Could you check a few things on this model? Use its own coordinates, in mm. Face numbers are marked on the shaded views. A direction names the side the tool comes from. Round coordinates to 2 decimals unless told otherwise and drop trailing zeros. Write each loop counter-clockwise with the first axis right and the second up, starting at its lowest first coordinate (ties: lowest second). Pieces come first, ordered by that corner, then holes. Notation, with made-up numbers: (82, 78.25) -> (134, 78.25) arc R24 cw to (134, 97.25) -> close; hole circle Ø5 at (-12.5, -18.5). An arc over 180 degrees is marked (long way). Answer as CSV lines item,"result". Start each with the question number.
Q1. If I drill on line 1 (Z direction, x = 37, y = 35); line 2 (X direction, y = 33, z = 1.5); line 3 (Y direction, x = 20, z = 3.75), over which ranges is the centre line in solid material (lowest first)? Write a range as [from, to].
Q2. Imagine slicing it at B-B on y = 26. Please give me the cut outline in (x, z), and give its area (3 significant figures).
Q3. For the marked faces 1 and 2, which set-ups out of +Z, -Z, +X, -X, +Y, -Y let a thin tool reach every point of the face, with its end or its side?
Q4. Imagine slicing it at A-A on z = 1.75. Please give me the cut outline in (x, y).
Q5. Imagine slicing it at D-D on y = 3. Please give me the cut outline in (x, z), and give its area (3 significant figures).
Q6. Will these pins go through, and if not, where does the flat tip stop? pin 1 Ø1 at (y, z) = (32, 5) entering from -X; pin 2 Ø1.2 at (x, y) = (38.87, 51.02) entering from +Z; pin 3 Ø2.5 at (x, z) = (5.5, 1) entering from -Y; pin 4 Ø3.5 at (y, z) = (46.5, 1.5) entering from -X.
Q7. Imagine slicing it at C-C on x = 12.5. Please give me the cut outline in (y, z), and give its area (3 significant figures).
from build123d import *

# Parameters (mm, degrees)
SKETCH1_R           = 17.265633628
SKETCH1_R_2         = 1
SKETCH1_R_3         = 10
SKETCH1_W           = 25
SKETCH1_H           = 3
BOSS_EXTRUDE5_DEPTH = 3
SKETCH2_R           = 17.5
BOSS_EXTRUDE6_DEPTH = 6.5


with BuildPart() as part:
    # Sketch1 → Boss-Extrude5 (new body)
    # profile 1 of 3: a face of its own
    with BuildSketch(Plane.XY):
        with BuildLine():
            Line((0, 0), (7.5, 0))
            Line((7.5, 0), (32.5, 0))
            Line((32.5, 0), (40, 0))
            Line((40, 0), (40, 6.867081787))
            ThreePointArc((40, 6.867081787), (43.887871625, 14.125845764), (45.231531638, 22.249870507))
            Line((45.231531638, 22.249870507), (45.231531638, 51.023857348))
            ThreePointArc((45.231531638, 51.023857348), (38.865765819, 57.389623167), (32.5, 51.023857348))
            Line((32.5, 51.023857348), (32.5, 44.167447672))
            ThreePointArc((32.5, 44.167447672), (0.97654543, 38.82510399), (0, 6.867081787))
            Line((0, 6.867081787), (0, 0))
        make_face()
        with Locations((20, 22.249870507)):
            Circle(SKETCH1_R, mode=Mode.SUBTRACT)
        with Locations((38.865765819, 51.023857348)):
            Circle(SKETCH1_R_2, mode=Mode.SUBTRACT)
    # profile 2 of 3: a face of its own
    with BuildSketch(Plane.XY):
        with Locations((20, 22.249870507)):
            Circle(SKETCH1_R)
        with Locations((20, 22.249870507)):
            Circle(SKETCH1_R_3, mode=Mode.SUBTRACT)
    # profile 3 of 3: a face of its own
    with BuildSketch(Plane.XY):
        with Locations((20, -1.5)):
            Rectangle(SKETCH1_W, SKETCH1_H)
    extrude(amount=BOSS_EXTRUDE5_DEPTH)

    # Sketch2 → Boss-Extrude6 (add)
    with BuildSketch(Plane(origin=(0, 0, 0), x_dir=(-1, 0, 0), z_dir=(0, 0, -1))):
        with Locations((-20, 22.249870507)):
            Circle(SKETCH2_R)
    extrude(amount=-BOSS_EXTRUDE6_DEPTH)


solid = part.part
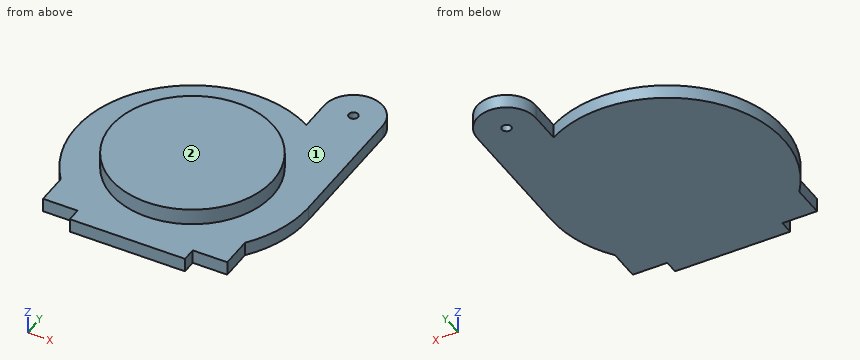
Checks:
1,line 1,"[0, 3]"
1,line 2,"[-2.83, 45.23]"
1,line 3,"[4.75, 39.75]"
2,outline,"(-4.95, 0) -> (45.23, 0) -> (45.23, 3) -> (37.09, 3) -> (37.09, 6.5) -> (2.91, 6.5) -> (2.91, 3) -> (-4.95, 3) -> close"
2,area,"270 mm^2"
3,face 1,"+Z"
3,face 2,"+Z, +X, -X, +Y, -Y"
4,outline,"(0, 0) -> (7.5, 0) -> (7.5, -3) -> (32.5, -3) -> (32.5, 0) -> (40, 0) -> (40, 6.87) arc R25.23 ccw to (45.23, 22.25) -> (45.23, 51.02) arc R6.37 ccw to (32.5, 51.02) -> (32.5, 44.17) arc R25.23 ccw to (0, 6.87) -> close; hole circle Ø2 at (38.87, 51.02)"
5,outline,"(0, 0) -> (40, 0) -> (40, 3) -> (0, 3) -> close"
5,area,"120 mm^2"
6,pin 1,"x = 5.14"
6,pin 2,"through"
6,pin 3,"y = 0"
6,pin 4,"x = 8.58"
7,outline,"(-3, 0) -> (46.34, 0) -> (46.34, 3) -> (38.06, 3) -> (38.06, 6.5) -> (6.44, 6.5) -> (6.44, 3) -> (-3, 3) -> close"
7,area,"259 mm^2"
